from build123d import *

# Parameters (mm, degrees)
F0_W     = 4.6
F0_H     = 10
F0_W_2   = 10
F0_H_2   = 4.75
F0_H_3   = 4.65
F0_W_3   = 4.7
F1_DEPTH = 10
F3_DEPTH = 5


with BuildPart() as f1:
    # F0 (on Top) → F1 (new body)
    with BuildSketch(Plane.XY):
        Polygon((5.4, 0), (0, 0), (0, -5.25), (0, -10), (0, -14.75), (0, -20), (5.3, -20), (10, -20), (14.7, -20), (20, -20), (20, -14.65), (20, -10), (20, -5.35), (20, 0), (14.6, 0), (10, 0), align=None)
        with Locations((7.7, 5)):
            Rectangle(F0_W, F0_H)
        with Locations((-5, -7.625)):
            Rectangle(F0_W_2, F0_H_2)
        with Locations((12.3, 5)):
            Rectangle(F0_W, F0_H)
        with Locations((-5, -12.375)):
            Rectangle(F0_W_2, F0_H_2)
        with Locations((25, -7.675)):
            Rectangle(F0_W_2, F0_H_3)
        with Locations((7.65, -25)):
            Rectangle(F0_W_3, F0_H)
        with Locations((25, -12.325)):
            Rectangle(F0_W_2, F0_H_3)
        with Locations((12.35, -25)):
            Rectangle(F0_W_3, F0_H)
    extrude(amount=F1_DEPTH)

    # F2 (on face) → F3 (cut)
    with BuildSketch(Plane.XY.offset(10)):
        Polygon((4.301277, -14.728494), (10, -14.7), (9.949831, -4.666128), align=None)
    extrude(amount=-F3_DEPTH, mode=Mode.SUBTRACT)


solid = f1.part
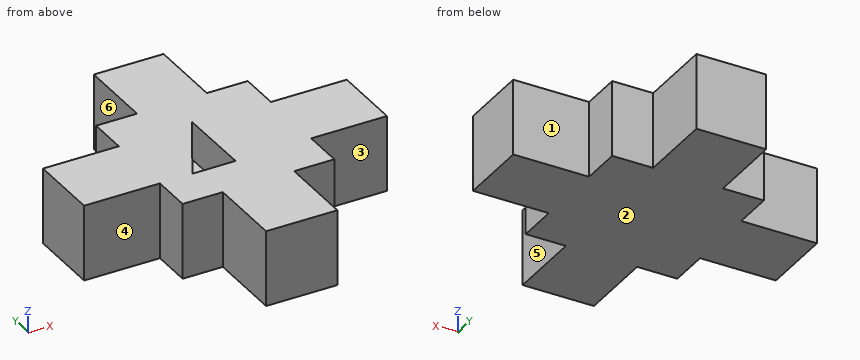
Verification items for the finished model (mm, model axes). Face numbers are marked on the shaded views. A direction names the side the tool comes from. Coordinates: 2 decimals unless noted, no trailing zeros. Order: outer loops, then holes, each group sorted by start corner. A loop starts at its lowest first (then second) coordinate and runs counter-clockwise, first axis right, second up. Notation, with made-up numbers: M 25.5,-31.5 L 44.5,-31.5 A15 cw 44.5,-12.5 Z; hole C 31,25 d11. An arc over 180 degrees is marked long. One line per item, written item: value. Start each with the question number.
Item 1: Gauge pin test, flat ends, axial feed: pin 1 (3 mm diameter, centred on y = -26.5, z = 3, fed in from -X); pin 2 (5 mm diameter, centred on x = 23.5, z = 6.5, fed in from +Y); pin 3 (1.5 mm diameter, centred on x = 17, z = 3, fed in from -Y). Record the tip position at first contact, or that the pin passes through.
Item 2: Sectioned sample at A-A (z = 7). Enter the section's corners in (x, y).
Item 3: Sectioned sample at B-B (x = -1). Enter the section's corners in (y, z), then the cut area to 3 significant figures.
Item 4: Mould release check, pull along Y, two halves, no side actions. Record for the marked faces 1, 2 and 3: released by +Y, released by -Y, zero draft, split by the parting line, or undercut.
Item 5: Access from +Z, -Z, +X, -X, +Y, -Y to the whole of each face (thin tool, end or side, straight path). Record for the marked faces 4, 5 and 6.
Item 6: Sectioned sample at D-D (z = 4). Enter the section's corners in (x, y), then the cut area to 3 significant figures.
Item 7: Sectioned sample at C-C (y = -26). Enter the section's corners in (x, z).
Item 8: Scan lines: probe 1 along X at (y, z) = (-18.5, 4); probe 2 along X at (y, z) = (-22, 4.25); probe 3 along Y at (x, z) = (-5, 7.75). Record each from-to range of solid material in increasing order.
Conclusion:
1. pin 1: stops at x = 5.3
1. pin 2: stops at y = -5.35
1. pin 3: stops at y = -20
2. outline: M -10,-14.75 L 0,-14.75 L 0,-20 L 5.3,-20 L 5.3,-30 L 14.7,-30 L 14.7,-20 L 20,-20 L 20,-14.65 L 30,-14.65 L 30,-5.35 L 20,-5.35 L 20,0 L 14.6,0 L 14.6,10 L 5.4,10 L 5.4,0 L 0,0 L 0,-5.25 L -10,-5.25 Z; hole M 4.3,-14.73 L 10,-14.7 L 9.95,-4.67 Z
3. outline: M -14.75,0 L -5.25,0 L -5.25,10 L -14.75,10 Z
3. area: 95.0 mm^2
4. face 1: released by +Y
4. face 2: zero draft
4. face 3: released by -Y
5. face 4: +Z, -Z, -X, -Y
5. face 5: +Z, -Z, +X, -Y
5. face 6: +Z, -Z, -X, +Y
6. outline: M -10,-14.75 L 0,-14.75 L 0,-20 L 5.3,-20 L 5.3,-30 L 14.7,-30 L 14.7,-20 L 20,-20 L 20,-14.65 L 30,-14.65 L 30,-5.35 L 20,-5.35 L 20,0 L 14.6,0 L 14.6,10 L 5.4,10 L 5.4,0 L 0,0 L 0,-5.25 L -10,-5.25 Z
6. area: 774 mm^2
7. outline: M 5.3,0 L 14.7,0 L 14.7,10 L 5.3,10 Z
8. probe 1: x = 0 to 20
8. probe 2: x = 5.3 to 14.7
8. probe 3: y = -14.75 to -5.25
